Here's how the part is built. I have some questions about the finished solid (model axes, mm). Face numbers are marked on the shaded views. A direction names the side the tool comes from. Round coordinates to 2 decimals unless told otherwise and drop trailing zeros. Order: outer loops, then holes, each group sorted by start corner. A loop starts at its lowest first (then second) coordinate and runs counter-clockwise, first axis right, second up. Notation, with made-up numbers: (-23.75, 29.5) - (4.25, 29.5) arc R16 ccw to (4.25, 54.5) - close; hole circle Ø7 at (25, 25). An arc over 180 degrees is marked (long way). One line per item, written item: value.
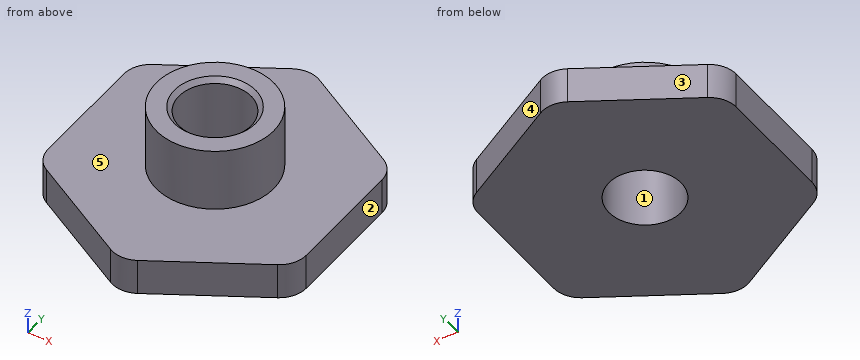
from build123d import *

# Parameters (mm, degrees)
SKETCH_R      = 4
PAD_DEPTH     = 4
SKETCH001_R   = 6.5
SKETCH001_R_2 = 4
PAD001_DEPTH  = 7
CHAMFER_SIZE  = 0.5
FILLET_R      = 3


with BuildPart() as part:
    # Sketch → Pad (new body)
    with BuildSketch(Plane.XY):
        Polygon((0, 16.5), (-14.289419, 8.25), (-14.289419, -8.25), (0, -16.5), (14.289419, -8.25), (14.289419, 8.25), align=None)
        Circle(SKETCH_R, mode=Mode.SUBTRACT)
    extrude(amount=PAD_DEPTH)

    # Sketch001 (on Face9 of Pad) → Pad001 (join)
    with BuildSketch(Plane.XY.offset(4)):
        Circle(SKETCH001_R)
        Circle(SKETCH001_R_2, mode=Mode.SUBTRACT)
    extrude(amount=PAD001_DEPTH)

    # Chamfer
    chamfer_edges = [part.edges().sort_by_distance(p)[0] for p in [
        (-4, 0, 11),
    ]]
    chamfer(chamfer_edges, length=CHAMFER_SIZE)

    # Fillet
    fillet_edges = [part.edges().sort_by_distance(p)[0] for p in [
        (0, -16.5, 2),
        (14.289419, -8.25, 2),
        (14.289419, 8.25, 2),
        (-14.289419, -8.25, 2),
        (-14.289419, 8.25, 2),
        (0, 16.5, 2),
    ]]
    fillet(fillet_edges, radius=FILLET_R)


solid = part.part
Q1. If we section it at A-A, the plane x = 0: Please give me the cut outline in (y, z).
Results list:
outline: (-16.04, 0) - (-4, 0) - (-4, 10.5) - (-4.5, 11) - (-6.5, 11) - (-6.5, 4) - (-16.04, 4) - close; (4, 0) - (16.04, 0) - (16.04, 4) - (6.5, 4) - (6.5, 11) - (4.5, 11) - (4, 10.5) - close
Q2. Will these pins go through, and if not, where does the flat tip stop? pin 1 (4 mm diameter, centred on x = 4.5, z = 5, fed in from -Y); pin 2 (10 mm diameter, centred on x = -5, y = -12, fed in from +Z); pin 3 (1.5 mm diameter, centred on x = 6, z = 6, fed in from -Y).
Results list:
pin 1: y = -14.9
pin 2: z = 4
pin 3: y = -3.83
Q3. If I drill on line 1 along Y through (x, z) = (0, 6); line 2 along Z through (x, y) = (-7, -12); line 3 along X through (y, z) = (2, 9.25), over which ranges is the centre line in solid material (lowest first)?
Results list:
line 1: -6.5 to -4, 4 to 6.5
line 2: 0 to 4
line 3: -6.18 to -3.46, 3.46 to 6.18
Q4. If we section it at C-C, the plane z = 6.5: Please give me the cut outline in (x, y).
Results list:
outline: circle Ø13 at (0, 0); hole circle Ø8 at (0, 0)
Q5. If we section it at B-B, the plane y = 0: Please give me the cut outline in (x, z).
Results list:
outline: (-14.29, 0) - (-4, 0) - (-4, 10.5) - (-4.5, 11) - (-6.5, 11) - (-6.5, 4) - (-14.29, 4) - close; (4, 0) - (14.29, 0) - (14.29, 4) - (6.5, 4) - (6.5, 11) - (4.5, 11) - (4, 10.5) - close
Q6. We'd pull the mould along X, two halves only. Please class the marked faces 1, 2 and 3: released by +X, released by -X, zero draft, split by the parting line, or undercut.
Results list:
face 1: undercut
face 2: released by +X
face 3: released by -X
Q7. If we section it at D-D, the plane y = 5: Please give me the cut outline in (x, z).
Results list:
outline: (-14.29, 0) - (14.29, 0) - (14.29, 4) - (4.15, 4) - (4.15, 11) - (-4.15, 11) - (-4.15, 4) - (-14.29, 4) - close
Q8. Which directions (+Z, -Z, +X, -X, +Y, -Y) give clear straight access to the entire face, cutting with the end or side of a thin tool? Please do the marked faces 4 and 5.
Results list:
face 4: +Z, -Z, +X, +Y
face 5: +Z
